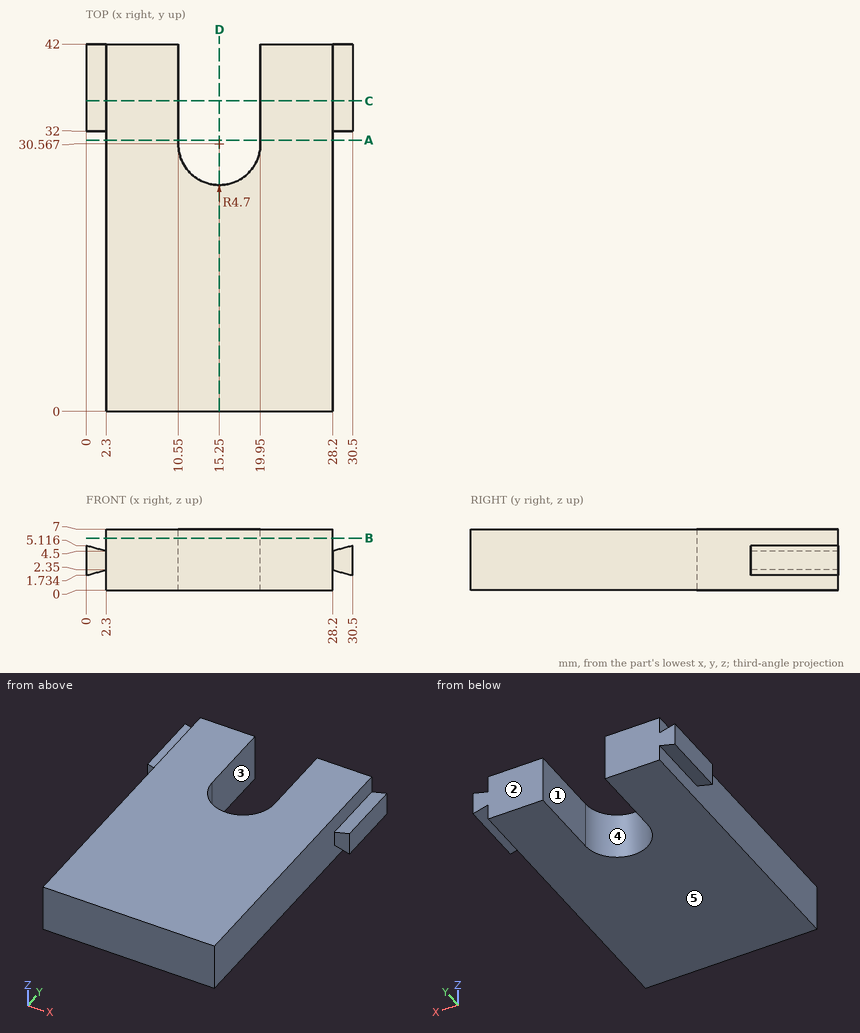
Source: three-view drawing plus pictorial views. Frame: mm from the lowest corner of the part. A direction names the side the tool comes from. Give positions to 0.01 mm unless a question says otherwise; leave off trailing zeros. Order: outer loops, then holes, each group sorted by start corner. A loop starts at its lowest first (then second) coordinate and runs counter-clockwise, first axis right, second up. Notation, with made-up numbers: M 45.25,35 L 70.25,35 A34 ccw 70.25,67 Z; hole C -31,-10 d6. An arc over 180 degrees is marked long. One line per question, with ' | ' between items.
1) Section C-C on y = 35.5. Output: boundary loops of the cut face in (x, z), and give its area (3 significant figures).
Filled in:
outline: M 0,1.73 L 2.3,2.35 L 2.3,0 L 10.55,0 L 10.55,7 L 2.3,7 L 2.3,4.5 L 0,5.12 Z; M 19.95,0 L 28.2,0 L 28.2,2.35 L 30.5,1.73 L 30.5,5.12 L 28.2,4.5 L 28.2,7 L 19.95,7 Z | area: 128 mm2
2) Section A-A on y = 31. Output: boundary loops of the cut face in (x, z), and give its area (4 significant figures).
Filled in:
outline: M 2.3,0 L 10.55,0 L 10.55,7 L 2.3,7 Z; M 19.95,0 L 28.2,0 L 28.2,7 L 19.95,7 Z | area: 115.5 mm2
3) Section B-B on z = 6. Output: boundary loops of the cut face in (x, y), and give its area (3 significant figures).
Filled in:
outline: M 2.3,0 L 28.2,0 L 28.2,42 L 19.95,42 L 19.95,30.57 A4.7 cw 10.55,30.57 L 10.55,42 L 2.3,42 Z | area: 946 mm2
4) Access query for the marked faces 1 and 2. Directions: +Z, -Z, +X, -X, +Y, -Y. A direction counts if a zero-diameter tool reaches every point of the face in a straight line with its end or side. Return the directions, or none.
Filled in:
face 1: +Z, -Z, +Y | face 2: +Z, -Z, +X, -X, +Y
5) Section D-D on x = 15.25. Output: boundary loops of the cut face in (y, z), and give its area (3 significant figures).
Filled in:
outline: M 0,0 L 25.87,0 L 25.87,7 L 0,7 Z | area: 181 mm2
6) Draft query along X for the marked faces 3, 4 and 5. Return one class per face: pulls with the +X half, pulls with the -X half, needs draft (parallel to the pull), parting line crosses it, or undercut.
Filled in:
face 3: undercut | face 4: undercut | face 5: needs draft
7) Contact query for flat-ended pins moving along their axis: P1, Ø2, axis at y = 37, z = 2, coming from the -X side; P2, Ø2, axis at y = 23, z = 3, coming from the -X side; P3, Ø0.7, axis at x = 1.5, z = 3, coming from the -Y side. Output: stop coordinate, or through.
Filled in:
P1: stops at x = 0 | P2: stops at x = 2.3 | P3: stops at y = 32
8) Ray query, L1, parallel to X at y = 32.5, z = 2.5; L2, parallel to X at y = 34, z = 6.5; L3, parallel to X at y = 25.5, z = 0.5. Return the intervals inside material, ascending.
Filled in:
L1: x = 0 to 10.55, 19.95 to 30.5 | L2: x = 2.3 to 10.55, 19.95 to 28.2 | L3: x = 2.3 to 28.2
